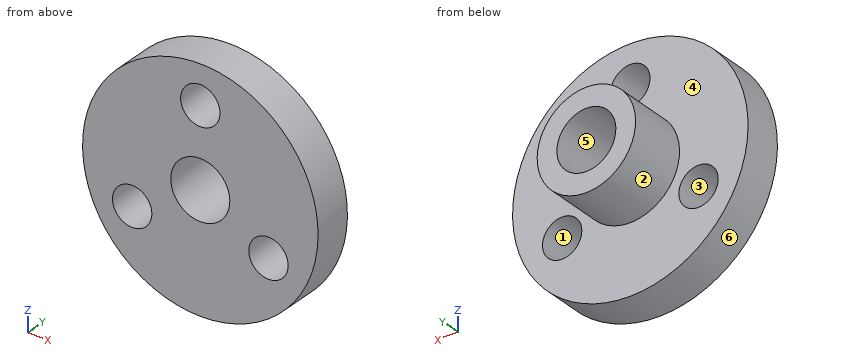
```python
from build123d import *

# Parameters (mm, degrees)
SKETCH1_R           = 9.5
BOSS_EXTRUDE1_DEPTH = 3.18
SKETCH2_R           = 3.97
BOSS_EXTRUDE2_DEPTH = 4.76
SKETCH3_R           = 2.38
CUT_EXTRUDE1_DEPTH  = 16.605883506
SKETCH4_R           = 1.5875
CUT_EXTRUDE2_DEPTH  = 15.253336452


with BuildPart() as part:
    # Sketch1 → Boss-Extrude1 (new body)
    with BuildSketch(Plane(origin=(0, 0, 0), x_dir=(1, 0, 0), z_dir=(0, 1, 0))):
        with Locations(Location((0, 0, 0), (0, 0, 90))):
            Circle(SKETCH1_R)
    extrude(amount=BOSS_EXTRUDE1_DEPTH)

    # Sketch2 → Boss-Extrude2 (add)
    with BuildSketch(Plane(origin=(0, 3.18, 0), x_dir=(1, 0, 0), z_dir=(0, 1, 0))):
        with Locations(Location((0, 0, 0), (0, 0, 270))):
            Circle(SKETCH2_R)
    extrude(amount=BOSS_EXTRUDE2_DEPTH)

    # Sketch3 → Cut-Extrude1 (cut, through all)
    with BuildSketch(Plane(origin=(0, 7.94, 0), x_dir=(1, 0, 0), z_dir=(0, 1, 0))):
        with Locations(Location((0, 0, 0), (0, 0, 270))):
            Circle(SKETCH3_R)
    extrude(amount=-CUT_EXTRUDE1_DEPTH, mode=Mode.SUBTRACT)

    # Sketch4 → Cut-Extrude2 (cut, through all)
    with BuildSketch(Plane(origin=(0, 3.18, 0), x_dir=(1, 0, 0), z_dir=(0, 1, 0))):
        with Locations(Location((0, -6.35, 0), (0, 0, 270))):
            Circle(SKETCH4_R)
        with Locations(Location((-5.499261314, 3.175, 0), (0, 0, 270))):
            Circle(SKETCH4_R)
        with Locations(Location((5.499261314, 3.175, 0), (0, 0, 270))):
            Circle(SKETCH4_R)
    extrude(amount=-CUT_EXTRUDE2_DEPTH, mode=Mode.SUBTRACT)


solid = part.part
```
Source: CAD feature listing. Evaluate the final solid. Frame: model axes, mm. Face numbers are marked on the shaded views. A direction names the side the tool comes from. Give positions to 0.01 mm unless a question says otherwise; leave off trailing zeros. Loops run counter-clockwise (first coordinate to the right, second up) from the corner with the lowest first, then second, coordinate; pieces in that order, holes last. Notation, with made-up numbers: M 27.25,51.25 L 38.25,51.25 A23 ccw 38.25,70.25 Z; hole C -24.5,-29 d11. An arc over 180 degrees is marked long. Put each result on its own line as item: value.
Q1. Pin query (flat end, axial travel): P1, Ø3.5, axis at x = 0, z = 6.35, coming from the -Y side; P2, Ø1.5, axis at y = 4.5, z = -2.5, coming from the -X side. Return the tip coordinate at first contact, or that it passes through.
Response values:
P1: stops at y = 0
P2: stops at x = -3.56
Q2. Section B-B (x = 0). Return the cut outline in (y, z).
Response values:
outline: M 0,-9.5 L 3.18,-9.5 L 3.18,-3.97 L 7.94,-3.97 L 7.94,-2.38 L 0,-2.38 Z; M 0,2.38 L 7.94,2.38 L 7.94,3.97 L 3.18,3.97 L 3.18,4.76 L 0,4.76 Z; M 0,7.94 L 3.18,7.94 L 3.18,9.5 L 0,9.5 Z
Q3. Section C-C (y = 4.5). Return the cut outline in (x, z), and give its area (3 significant figures).
Response values:
outline: C 0,0 d7.94; hole C 0,0 d4.76
area: 31.7 mm²
Q4. Reachability of the marked faces 1 and 2 from +Z, -Z, +X, -X, +Y, -Y: full face, straight path, thin tool, end or side. Return the list, or none.
Response values:
face 1: +Y, -Y
face 2: +Y
Q5. Section D-D (z = 6.25). Return the cut outline in (x, y).
Response values:
outline: M -7.15,0 L -1.58,0 L -1.58,3.18 L -7.15,3.18 Z; M 1.58,0 L 7.15,0 L 7.15,3.18 L 1.58,3.18 Z
Q6. Line query: probe 1 along X at (y, z) = (2, 0); probe 2 along X at (y, z) = (4.25, 0); probe 3 along Y at (x, z) = (5.75, 5.25). Output: solid intervals per line, ascending. Write a range as [from, to].
Response values:
probe 1: x = [-9.5, -2.38], [2.38, 9.5]
probe 2: x = [-3.97, -2.38], [2.38, 3.97]
probe 3: y = [0, 3.18]
Q7. Section A-A (z = 0). Return the cut outline in (x, y).
Response values:
outline: M -9.5,0 L -2.38,0 L -2.38,7.94 L -3.97,7.94 L -3.97,3.18 L -9.5,3.18 Z; M 2.38,0 L 9.5,0 L 9.5,3.18 L 3.97,3.18 L 3.97,7.94 L 2.38,7.94 Z
Q8. Mould query, pull axis Z, two halves, no side actions, for the marked faces 3, 4, 5 and 6. Classes: released by +Z, released by -Z, zero draft, split by the parting line, or undercut.
Response values:
face 3: undercut
face 4: zero draft
face 5: undercut
face 6: split by the parting line
